The drawing under review shows one solid part. Ordinate dimensions are in mm from its lowest x, y, z. A direction names the side the tool comes from. Give positions to 0.01 mm unless a question says otherwise; leave off trailing zeros. Order: outer loops, then holes, each group sorted by start corner. A loop starts at its lowest first (then second) coordinate and runs counter-clockwise, first axis right, second up. Notation, with made-up numbers: (88.25, 21) -> (147.25, 21) arc R18 ccw to (147.25, 46) -> close; hole circle Ø3 at (43, -6.5). An arc over 180 degrees is marked (long way). One line per item, written item: value.
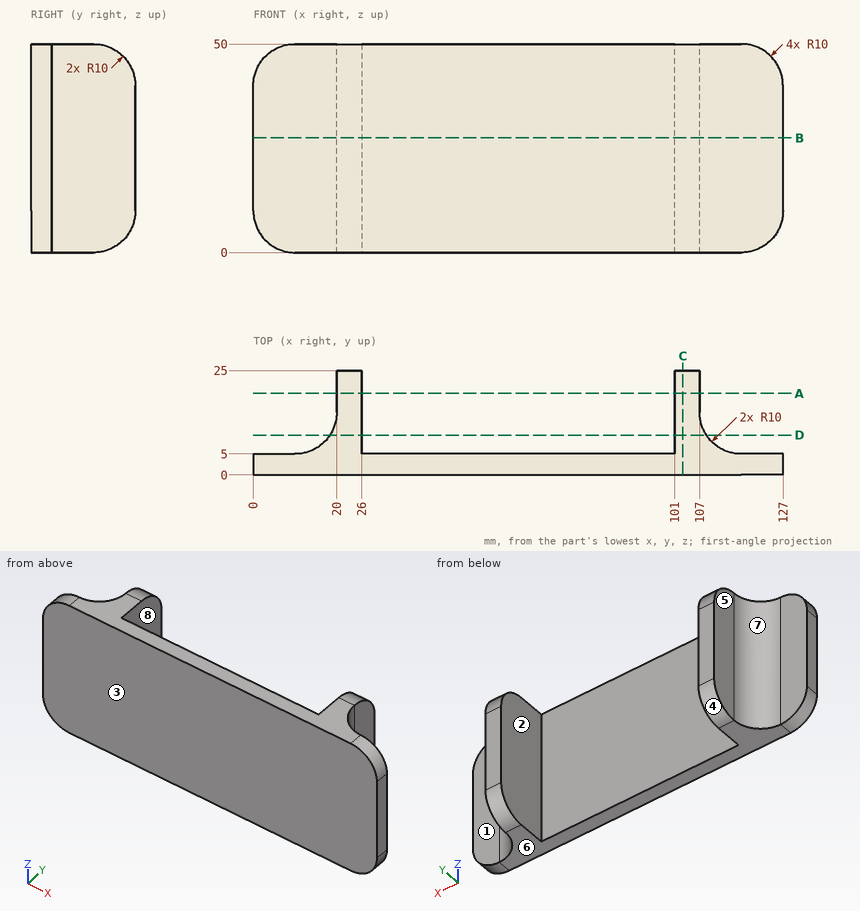
Item 1: Add section C-C on x = 103. Give the boundary of the cut face in (y, z).
Returned:
outline: (0, 0) -> (15, 0) arc R10 ccw to (25, 10) -> (25, 40) arc R10 ccw to (15, 50) -> (0, 50) -> close
Item 2: Add section D-D on y = 9.5. Give the boundary of the cut face in (x, z), plus the area to 3 significant figures.
Returned:
outline: (18.35, 0) -> (26, 0) -> (26, 50) -> (18.35, 50) -> close; (101, 0) -> (108.65, 0) -> (108.65, 50) -> (101, 50) -> close
area: 765 mm²
Item 3: Clearance check with flat-ended pins moving along their axes: P1, Ø6, axis at y = 19.5, z = 14, coming from the +X side; P2, Ø11, axis at y = 19.5, z = 17.5, coming from the +X side; P3, Ø1, axis at y = 13, z = 33.5, coming from the -X side. State where each tip first meets the part, or that it passes through.
Returned:
P1: x = 107
P2: x = 107.05
P3: x = 19.68
Item 4: Draft analysis for pull direction X (two halves, no side actions). For the marked faces 6, 7 and 8, state which applies: pulls with the +X half, pulls with the -X half, needs draft (parallel to the pull), parting line crosses it, or undercut.
Returned:
face 6: needs draft
face 7: pulls with the -X half
face 8: undercut
Item 5: Add section B-B on z = 27.5. Give the boundary of the cut face in (x, y).
Returned:
outline: (0, 0) -> (127, 0) -> (127, 5) -> (117, 5) arc R10 cw to (107, 15) -> (107, 25) -> (101, 25) -> (101, 5) -> (26, 5) -> (26, 25) -> (20, 25) -> (20, 15) arc R10 cw to (10, 5) -> (0, 5) -> close
Item 6: Add section A-A on y = 19.5. Give the boundary of the cut face in (x, z), plus the area to 3 significant figures.
Returned:
outline: (20, 1.07) -> (26, 1.07) -> (26, 48.93) -> (20, 48.93) -> close; (101, 1.07) -> (107, 1.07) -> (107, 48.93) -> (101, 48.93) -> close
area: 574 mm²
Item 7: To check wall thickness, follow line 1 along Y through (x, z) = (10, 21.5); line 2 along X through (y, z) = (17.5, 28); line 3 along X through (y, z) = (9.75, 36). State the ranges of each line that lie inside material, in increasing order. Write a range as from..to.
Returned:
line 1: 0..5
line 2: 20..26, 101..107
line 3: 18.51..26, 101..108.49
Item 8: Machinability: for the marked faces 1, 2, 3, 4 and 5, which of the approach directions +Z, -Z, +X, -X, +Y, -Y give a long, thin tool a straight path to every point of the face, cutting with its end or side? Answer none if there is none.
Returned:
face 1: +Z, -Z, +X, +Y
face 2: +Z, -Z, +Y
face 3: +Z, -Z, +X, -X, -Y
face 4: -Z, +X, -X, +Y
face 5: +Z, -Z, -X, +Y
